Job drawing, mm, ordinate dimensions from the low corner. One solid piece. A direction names the side the tool comes from. Give positions to 0.01 mm unless a question says otherwise; leave off trailing zeros. Write each loop counter-clockwise with the first axis right and the second up, starting at its lowest first coordinate (ties: lowest second). Pieces come first, ordered by that corner, then holes. Notation, with made-up numbers: (12.5, -10.5) -> (56.5, -10.5) arc R29 cw to (56.5, 14.5) -> close; hole circle Ø7 at (19.5, 0). An arc over 180 degrees is marked (long way). Put each result on its own line as item: value. Start each with the question number.
Item 1: Slice it at A-A, the plane x = 8. List the corners of the cut face in (y, z).
Item 2: Drill centre lines: line 1 along Z through (x, y) = (8, 14.7); line 2 along Z through (x, y) = (11.75, 2); line 3 along X through (y, z) = (8, 13.5). Where is each one in solid material? Low to high.
Item 3: Flat gauge pins, fed straight in: pin 1 Ø1 at (y, z) = (1.5, 5) entering from -X (1 decimal); pin 2 Ø6.5 at (x, z) = (8, 18.96) entering from +Y; pin 3 Ø1 at (y, z) = (10, 12) entering from -X. Where does each tip first touch, or does it go through?
Item 4: Two-plate mould, pull along Z, no slides. Class the marked faces 1, 2 and 3: pulls with the +Z half, pulls with the -Z half, needs draft (parallel to the pull), parting line crosses it, or undercut.
Item 5: Tool access for the marked faces 4 and 5: list every direction of +Z, -Z, +X, -X, +Y, -Y with a clear straight run to the whole face (end or side of a thin tool).
Item 6: Slice it at D-D, the plane x = 3.5. List the corners of the cut face in (y, z).
Item 7: Slice it at B-B, the plane y = 8. List the corners of the cut face in (x, z).
Item 8: Slice it at C-C, the plane z = 21.5. List the corners of the cut face in (x, y).
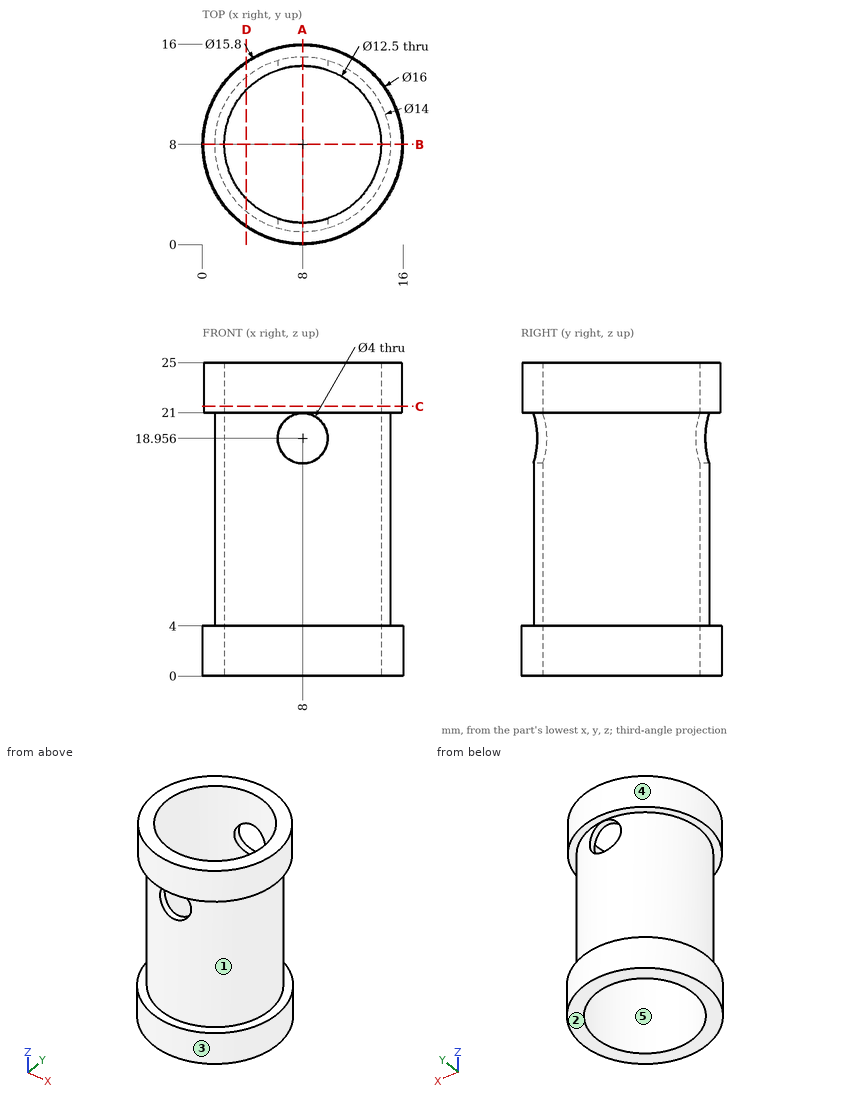
Values follow:
1. outline: (0, 0) -> (1.75, 0) -> (1.75, 16.96) -> (1, 16.96) -> (1, 4) -> (0, 4) -> close; (0.1, 21) -> (1, 21) -> (1, 20.96) -> (1.75, 20.96) -> (1.75, 25) -> (0.1, 25) -> close; (14.25, 0) -> (16, 0) -> (16, 4) -> (15, 4) -> (15, 16.96) -> (14.25, 16.96) -> close; (14.25, 20.96) -> (15, 20.96) -> (15, 21) -> (15.9, 21) -> (15.9, 25) -> (14.25, 25) -> close
2. line 1: 0 to 16.96, 20.96 to 25
2. line 2: 0 to 4, 21 to 25
2. line 3: 1 to 1.75, 14.25 to 15
3. pin 1: x = 4.4
3. pin 2: y = 15.9
3. pin 3: x = 1.16
4. face 1: undercut
4. face 2: pulls with the -Z half
4. face 3: needs draft
5. face 4: +Z
5. face 5: +Z, -Z
6. outline: (1.39, 0) -> (3.66, 0) -> (3.66, 25) -> (1.51, 25) -> (1.51, 21) -> (2.64, 21) -> (2.64, 4) -> (1.39, 4) -> close; (12.34, 0) -> (14.61, 0) -> (14.61, 4) -> (13.36, 4) -> (13.36, 21) -> (14.49, 21) -> (14.49, 25) -> (12.34, 25) -> close
7. outline: (0, 0) -> (1.75, 0) -> (1.75, 25) -> (0.1, 25) -> (0.1, 21) -> (1, 21) -> (1, 4) -> (0, 4) -> close; (14.25, 0) -> (16, 0) -> (16, 4) -> (15, 4) -> (15, 21) -> (15.9, 21) -> (15.9, 25) -> (14.25, 25) -> close
8. outline: circle Ø15.8 at (8, 8); hole circle Ø12.5 at (8, 8)
